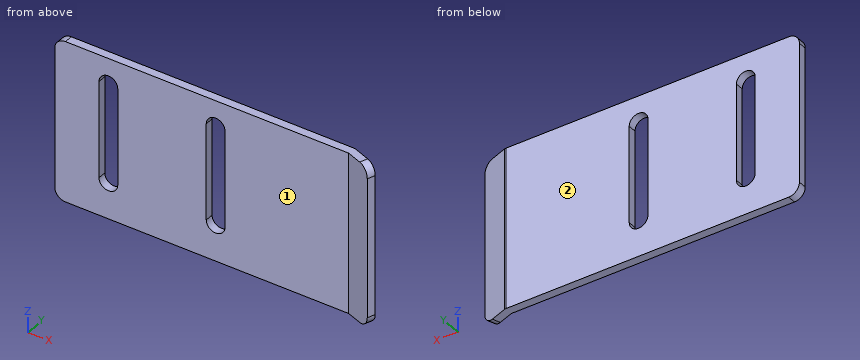
```python
from build123d import *

# Parameters (mm, degrees)
BOSS_EXTRUDE1_DEPTH = 30
FILLET1_R           = 1
FILLET2_R           = 2
CUT_EXTRUDE1_DEPTH  = 4.256447705


with BuildPart() as part:
    # Sketch1 → Boss-Extrude1 (new body)
    with BuildSketch(Plane.XY):
        Polygon((-37.577345781, 8.579229267), (17.308314067, 8.579229267), (22.382654219, 6.732320493), (21.869624004, 5.322781562), (17.222654219, 7.014140243), (-37.577345781, 7.014140243), align=None)
    extrude(amount=BOSS_EXTRUDE1_DEPTH)

    # Fillet1
    fillet1_edges = [part.edges().sort_by_distance(p)[0] for p in [
        (17.308314067, 8.579229267, 15),
    ]]
    fillet(fillet1_edges, radius=FILLET1_R)

    # Fillet2
    fillet2_edges = [part.edges().sort_by_distance(p)[0] for p in [
        (22.126139112, 6.027551028, 30),
        (-37.577345781, 7.796684755, 30),
        (22.126139112, 6.027551028, 0),
        (-37.577345781, 7.796684755, 0),
    ]]
    fillet(fillet2_edges, radius=FILLET2_R)

    # Sketch3 → Cut-Extrude1 (cut, through all)
    with BuildSketch(Plane(origin=(0, 8.579229267, 0), x_dir=(1, 0, 0), z_dir=(0, 1, 0))):
        with BuildLine():
            Line((-25.827345781, -25), (-25.827345781, -7))
            ThreePointArc((-25.827345781, -7), (-27.577345781, -5.25), (-29.327345781, -7))
            Line((-29.327345781, -7), (-29.327345781, -25))
            ThreePointArc((-29.327345781, -25), (-27.577345781, -26.75), (-25.827345781, -25))
        make_face()
        with BuildLine():
            Line((-5.827345781, -25), (-5.827345781, -7))
            ThreePointArc((-5.827345781, -7), (-7.577345781, -5.25), (-9.327345781, -7))
            Line((-9.327345781, -7), (-9.327345781, -25))
            ThreePointArc((-9.327345781, -25), (-7.577345781, -26.75), (-5.827345781, -25))
        make_face()
    extrude(amount=-CUT_EXTRUDE1_DEPTH, mode=Mode.SUBTRACT)


solid = part.part
```
Verification items for the finished model (mm, model axes). Face numbers are marked on the shaded views. A direction names the side the tool comes from. Give positions to 0.01 mm unless a question says otherwise; leave off trailing zeros. Order: outer loops, then holes, each group sorted by start corner. A loop starts at its lowest first (then second) coordinate and runs counter-clockwise, first axis right, second up. Notation, with made-up numbers: (33, 57) -> (48, 57) arc R22 cw to (48, 64) -> close; hole circle Ø9 at (2, 11). An arc over 180 degrees is marked (long way). Use a Markdown table: item, result.
1) Depth check by flat-ended pin: pin 1 Ø1.5 at (x, z) = (-4.5, 5) entering from -Y. Enter the tip coordinate at first touch or a pass-through.
Results:
| item | result |
|---|---|
| pin 1 | y = 7.01 |
2) Material ranges on probe 1 along Y at (x, z) = (-2, 4); probe 2 along Z at (x, y) = (20.5, 6.7), recorded low to high.
Results:
| item | result |
|---|---|
| probe 1 | 7.01 to 8.58 |
| probe 2 | 0.01 to 29.99 |
3) Tool access check on the marked faces 1 and 2. Record the directions out of +Z, -Z, +X, -X, +Y, -Y that give a thin tool (end or side, any length) a straight path to the whole face; none if there is none.
Results:
| item | result |
|---|---|
| face 1 | +Z, -Z, -X, -Y |
| face 2 | +Z, -Z, +X, -X, +Y |
4) Section check C-C, the plane x = 0.5. Record the boundary of the cut face in (y, z), then the cut area to 3 significant figures.
Results:
| item | result |
|---|---|
| outline | (7.01, 0) -> (8.58, 0) -> (8.58, 30) -> (7.01, 30) -> close |
| area | 47.0 mm² |
5) Section check D-D, the plane z = 26. Record the boundary of the cut face in (x, y).
Results:
| item | result |
|---|---|
| outline | (-37.58, 7.01) -> (-29.01, 7.01) -> (-29.01, 8.58) -> (-37.58, 8.58) -> close; (-26.14, 7.01) -> (-9.01, 7.01) -> (-9.01, 8.58) -> (-26.14, 8.58) -> close; (-6.14, 7.01) -> (17.22, 7.01) -> (21.87, 5.32) -> (22.38, 6.73) -> (17.47, 8.52) arc R1 ccw to (17.13, 8.58) -> (-6.14, 8.58) -> close |
6) Section check A-A, the plane z = 9.5. Record the boundary of the cut face in (x, y), then the cut area to 3 significant figures.
Results:
| item | result |
|---|---|
| outline | (-37.58, 7.01) -> (-29.33, 7.01) -> (-29.33, 8.58) -> (-37.58, 8.58) -> close; (-25.83, 7.01) -> (-9.33, 7.01) -> (-9.33, 8.58) -> (-25.83, 8.58) -> close; (-5.83, 7.01) -> (17.22, 7.01) -> (21.87, 5.32) -> (22.38, 6.73) -> (17.47, 8.52) arc R1 ccw to (17.13, 8.58) -> (-5.83, 8.58) -> close |
| area | 82.6 mm² |
7) Section check B-B, the plane z = 3.25. Record the boundary of the cut face in (x, y).
Results:
| item | result |
|---|---|
| outline | (-37.58, 7.01) -> (17.22, 7.01) -> (21.87, 5.32) -> (22.38, 6.73) -> (17.47, 8.52) arc R1 ccw to (17.13, 8.58) -> (-37.58, 8.58) -> close |
